Autodesk Inventor part; units mm, degrees
ref_plane "YZ Plane" through (0, 0, 0) normal (1, 0, 0) x (0, 1, 0)
ref_plane "XZ Plane" through (0, 0, 0) normal (0, 1, 0) x (-1, 0, 0)
ref_plane "XY Plane" through (0, 0, 0) normal (0, 0, 1) x (1, 0, 0)
sketch "Sketch1" plane through (0, 0, 0) normal (0, 0, 1) x (1, 0, 0)
  line L0 (0, 0) -> (-11.1125, 0) construction
  line L1 (0, 0) -> (0, 11.1125) construction
  line L2 (-11.1125, 11.1125) -> (11.1125, 11.1125)
  line L3 (11.1125, 11.1125) -> (11.1125, -11.1125)
  line L4 (11.1125, -11.1125) -> (-11.1125, -11.1125)
  line L5 (-11.1125, -11.1125) -> (-11.1125, 11.1125)
  line L6 (-12.7, 12.7) -> (12.7, 12.7)
  line L7 (12.7, 12.7) -> (12.7, -12.7)
  line L8 (12.7, -12.7) -> (-12.7, -12.7)
  line L9 (-12.7, -12.7) -> (-12.7, 12.7)
  line L10 (-11.1125, 0) -> (-12.7, 0) construction
  line L11 (0, 11.1125) -> (0, 12.7) construction
  dimension "d0" = 25.4
  dimension "d1" = 1.5875
extrude "Extrusion1" add sketch "Sketch1" along normal blind 330.2
sketch "Sketch2" plane through (12.7, -12.7, 0) normal (1, 0, 0) x (0, 0, -1)
  line L0 (0, 12.7) -> (-330.2, 12.7) construction
  line L1 (-330.2, 1.5875) -> (-330.2, 23.8125) construction
  circle A0 centre (-320.675, 12.7) radius 1.27
  circle A1 centre (-301.625, 12.7) radius 1.27
  circle A2 centre (-9.525, 12.7) radius 1.5875
  circle A3 centre (-28.575, 12.7) radius 1.5875
  dimension "d4" = 2.54
  dimension "d5" = 19.05
  dimension "d6" = 9.525
  dimension "d7" = 3.175
  dimension "d8" = 19.05
  dimension "d9" = 9.525
extrude "Extrusion2" cut sketch "Sketch2" against normal through all
sketch "Sketch3" plane through (-12.7, -12.7, 0) normal (0, -1, 0) x (1, 0, 0)
  circle A0 centre (12.7, 127) radius 1.5875
  circle A1 centre (12.7, 101.6) radius 1.5875
  line L0 (0, 0) -> (25.4, 0) construction
  line L1 (12.7, 0) -> (12.7, 101.6) construction
  line L2 (12.7, 101.6) -> (12.7, 127) construction
  line L3 (12.7, 114.3) -> (0, 114.3) construction
  line L4 (1.5875, 0) -> (1.5875, 330.2) construction
  dimension "d12" = 3.175
  dimension "d13" = 114.3
  dimension "d14" = 25.4
extrude "Extrusion3" cut sketch "Sketch3" against normal through all
properties part number "Short Side" material "Aluminum 6061"
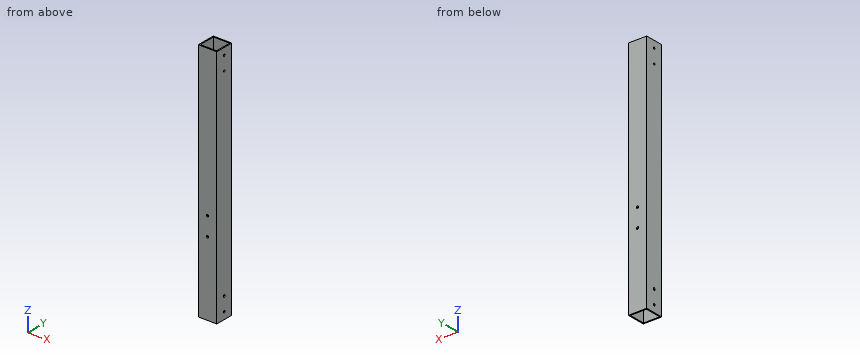
Design review of the part built by this model. Coordinates are the model's own, in mm. Coordinates: 2 decimals unless noted, no trailing zeros. Order: outer loops, then holes, each group sorted by start corner. A loop starts at its lowest first (then second) coordinate and runs counter-clockwise, first axis right, second up. Notation, with made-up numbers: (44, 63) - (64, 63) arc R15 ccw to (64, 75) - close; hole circle Ø3 at (2.5, 69.5). An arc over 180 degrees is marked (long way). One line per question, with ' | ' between items.
Q1. Consider section B-B, the plane z = 165. Give the boundary of the cut face in (x, y), then the cut area to 3 significant figures.
Answer key:
outline: (-12.7, -12.7) - (12.7, -12.7) - (12.7, 12.7) - (-12.7, 12.7) - close; hole (-11.11, -11.11) - (11.11, -11.11) - (11.11, 11.11) - (-11.11, 11.11) - close | area: 151 mm2
Q2. Consider section A-A, the plane x = -6.25. Give the boundary of the cut face in (y, z), then the cut area to 3 significant figures.
Answer key:
outline: (-12.7, 0) - (-11.11, 0) - (-11.11, 330.2) - (-12.7, 330.2) - close; (11.11, 0) - (12.7, 0) - (12.7, 330.2) - (11.11, 330.2) - close | area: 1,050 mm2
Q3. To check wall thickness, follow line 1 along Z through (x, y) = (0, -12.3); line 2 along Y through (x, z) = (-7.5, 18.5). State the ranges of each line that lie inside material, in increasing order.
Answer key:
line 1: z = 0 to 100.01, 103.19 to 125.41, 128.59 to 330.2 | line 2: y = -12.7 to -11.11, 11.11 to 12.7
